Geometry: see drawing. Coordinates: mm, zero at the bounding-box minimum. Give positions to 0.01 mm unless a question says otherwise; leave off trailing zeros. Write each loop counter-clockwise with the first axis right and the second up, starting at its lowest first coordinate (ties: lowest second). Pieces come first, ordered by that corner, then holes. Notation, with made-up numbers: (79.25, 57) - (84.25, 57) arc R13 ccw to (84.25, 72) - close; hole circle Ø9 at (-8, 62.5). An arc over 180 degrees is marked (long way). Use a Markdown table: item, result. Add a question column.
1. Mould query, pull axis X, two halves, no side actions, for the marked faces 1, 2 and 3. Classes: released by +X, released by -X, zero draft, split by the parting line, or undercut.
2. Pin query (flat end, axial travel): pin 1 (5 mm diameter, centred on y = 18, z = 29.5, fed in from -X); pin 2 (9 mm diameter, centred on x = 35, z = 30, fed in from -Y). Return the tip coordinate at first contact, or that it passes through.
3. Section query A-A, the plane x = 70. Return loops of the section in (y, z) (1 decimal).
4. Section query B-B, the plane z = 30. Return loops of the section in (x, y) (1 decimal), plus the area to 3 significant figures.
5. Material intervals for probe 1 along Z at (x, y) = (70, 13.25) (1 decimal); probe 2 along X at (y, z) = (9.5, 32.5); probe 3 along X at (y, z) = (17, 24), sorted ascending.
6. Section query C-C, the plane y = 10.5. Return loops of the section in (x, z) (1 decimal), plus the area to 3 significant figures.
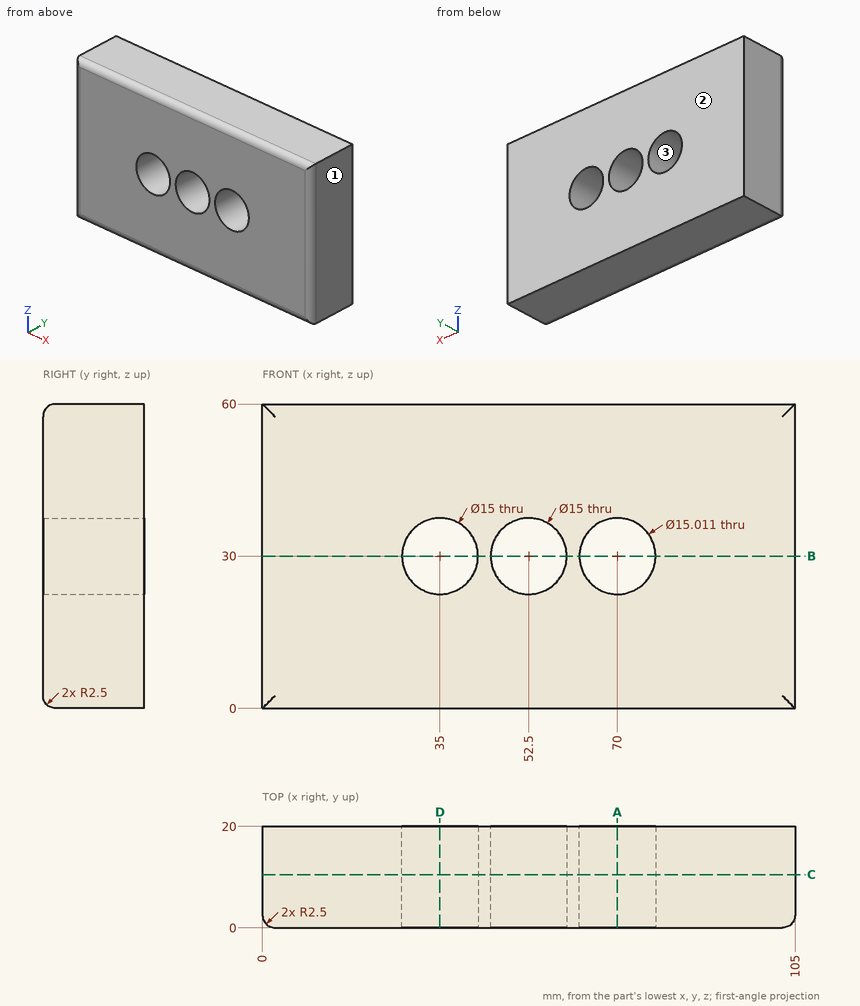
Result sheet:
| question | item | result |
|---|---|---|
| 1 | face 1 | released by +X |
| 1 | face 2 | zero draft |
| 1 | face 3 | undercut |
| 2 | pin 1 | stops at x = 0 |
| 2 | pin 2 | passes through |
| 3 | outline | (0, 2.5) arc R2.5 ccw to (2.5, 0) - (20, 0) - (20, 22.5) - (0, 22.5) - close; (0, 37.5) - (20, 37.5) - (20, 60) - (2.5, 60) arc R2.5 ccw to (0, 57.5) - close |
| 4 | outline | (0, 2.5) arc R2.5 ccw to (2.5, 0) - (27.5, 0) - (27.5, 20) - (0, 20) - close; (42.5, 0) - (45, 0) - (45, 20) - (42.5, 20) - close; (60, 0) - (62.5, 0) - (62.5, 20) - (60, 20) - close; (77.5, 0) - (102.5, 0) arc R2.5 ccw to (105, 2.5) - (105, 20) - (77.5, 20) - close |
| 4 | area | 1,200 mm² |
| 5 | probe 1 | z = 0 to 22.5, 37.5 to 60 |
| 5 | probe 2 | x = 0 to 27.93, 42.07 to 45.43, 59.57 to 62.92, 77.08 to 105 |
| 5 | probe 3 | x = 0 to 30.5, 39.5 to 48, 57 to 65.49, 74.51 to 105 |
| 6 | outline | (0, 0) - (105, 0) - (105, 60) - (0, 60) - close; hole circle Ø15 at (35, 30); hole circle Ø15 at (52.5, 30); hole circle Ø15 at (70, 30) |
| 6 | area | 5,770 mm² |
